from build123d import *

# Parameters (mm, degrees)
BOSS_EXTRUDE1_DEPTH = 0.64


with BuildPart() as part:
    # Sketch1 → Boss-Extrude1 (new body)
    with BuildSketch(Plane(origin=(0, 0, 0), x_dir=(1, 0, 0), z_dir=(0, 1, 0))):
        with BuildLine():
            Line((-1.112579474, 3.633478624), (-0.249511241, 1.782622826))
            ThreePointArc((-0.249511241, 1.782622826), (0, 1.8), (0.249511241, 1.782622826))
            Line((0.249511241, 1.782622826), (1.112579474, 3.633478624))
            ThreePointArc((1.112579474, 3.633478624), (2.774739275, 2.596309295), (3.699307386, 0.868979208))
            ThreePointArc((3.699307386, 0.868979208), (3.784949165, 0.337875445), (3.794733192, -0.2))
            Line((3.794733192, -0.2), (2.794733192, -0.2))
            Line((2.794733192, -0.2), (2.151945583, -0.966044443))
            Line((2.151945583, -0.966044443), (2.57594692, -3.370675522))
            Line((2.57594692, -3.370675522), (2.577455967, -3.37923375))
            ThreePointArc((2.577455967, -3.37923375), (0, 4.25), (-2.577455967, -3.37923375))
            Line((-2.577455967, -3.37923375), (-2.576768139, -3.375332886))
            Line((-2.576768139, -3.375332886), (-2.151945583, -0.966044443))
            Line((-2.151945583, -0.966044443), (-2.794733192, -0.2))
            Line((-2.794733192, -0.2), (-3.794733192, -0.2))
            ThreePointArc((-3.794733192, -0.2), (-3.784949165, 0.337875445), (-3.699307386, 0.868979208))
            ThreePointArc((-3.699307386, 0.868979208), (-2.774739275, 2.596309295), (-1.112579474, 3.633478624))
        make_face()
    extrude(amount=BOSS_EXTRUDE1_DEPTH)


solid = part.part
Design review of the part built by this model. Coordinates are the model's own, in mm. A direction names the side the tool comes from. Coordinates: 2 decimals unless noted, no trailing zeros. Loops run counter-clockwise (first coordinate to the right, second up) from the corner with the lowest first, then second, coordinate; pieces in that order, holes last. Notation, with made-up numbers: M -23,-18.5 L 26,-18.5 A20 cw 26,-13.5 Z; hole C -27.5,15.25 d2. An arc over 180 degrees is marked long. Answer as CSV lines item,"result".
Item 1: Add section C-C on x = 0. State the section outline as (y, z) points, plus the area to 3 significant figures.
Answer list:
outline,"M 0,-4.25 L 0.64,-4.25 L 0.64,-1.8 L 0,-1.8 Z"
area,"1.57 mm²"
Item 2: Add section D-D on x = -2. State the section outline as (y, z) points.
Answer list:
outline,"M 0,-3.75 L 0.64,-3.75 L 0.64,-3.23 L 0,-3.23 Z"
Item 3: Machinability: for faces 4 (the face through (0, 0.64, -2)), 5 (the face through (-0.687, 0.316, -2.721)), which of the approach directions +Z, -Z, +X, -X, +Y, -Y give a long, thin tool a straight path to every point of the face, cutting with its end or side? Answer none if there is none.
Answer list:
face 4,"+Z, -Z, +X, -X, +Y"
face 5,"+Z, +Y, -Y"
Item 4: For probe 1 along X at (y, z) = (0.35, -3); probe 2 along X at (y, z) = (0.3, -2.5); probe 3 along X at (y, z) = (0.15, 0.5), list the stretches that pass through material, from the lowest coordinate up.
Answer list:
probe 1,"-3.01 to -2.33, -0.82 to 0.82, 2.33 to 3.01"
probe 2,"-3.44 to -2.86, -0.58 to 0.58, 2.86 to 3.44"
probe 3,"-4.22 to -2.54, 2.54 to 4.22"
Item 5: For P1, Ø4, axis at x = 0.5, z = -1, coming from the -Y side, flat-tipped, find the tip position at first contact; note if it passes through.
Answer list:
P1,"y = 0"
Item 6: Add section A-A on z = 0. State the section outline as (x, y) points, plus the area to 3 significant figures.
Answer list:
outline,"M -4.25,0 L -3.8,0 L -3.8,0.64 L -4.25,0.64 Z; M 3.8,0 L 4.25,0 L 4.25,0.64 L 3.8,0.64 Z"
area,"0.576 mm²"
Item 7: The part is to be moulded in two halves that separate along X. For faces 1 (the face through (0.148, 0.316, -4.247)), 2 (the face through (0.675, 0.316, -2.695)), 3 (the face through (0, 0, -2)), say which applies: pulls with the +X half, pulls with the -X half, needs draft (parallel to the pull), parting line crosses it, or undercut.
Answer list:
face 1,"parting line crosses it"
face 2,"undercut"
face 3,"needs draft"
